Autodesk Inventor part; units mm, degrees
ref_plane "YZ Plane" through (0, 0, 0) normal (1, 0, 0) x (0, 1, 0)
ref_plane "XZ Plane" through (0, 0, 0) normal (0, 1, 0) x (-1, 0, 0)
ref_plane "XY Plane" through (0, 0, 0) normal (0, 0, 1) x (1, 0, 0)
sketch "Sketch1" plane through (0, 0, 0) normal (0, 0, 1) x (1, 0, 0)
  circle A0 centre (0, 0) radius 30
  dimension "d0" = 60
extrude "Extrusion1" add sketch "Sketch1" along normal mid plane 10
sketch "Sketch2" plane through (0, 0, 5) normal (0, 0, 1) x (1, 0, 0)
  circle A0 centre (0, 0) radius 30
  circle A1 centre (0, 0) radius 10
  dimension "d3" = 20
extrude "Extrusion2" add sketch "Sketch2" along normal blind 20 contours A1
sketch "Sketch3" plane through (0, 0, 25) normal (0, 0, 1) x (1, 0, 0)
  circle A0 centre (0, 0) radius 10
  circle A1 centre (0, 0) radius 5
  dimension "d6" = 10
extrude "Extrusion3" cut sketch "Sketch3" against normal through all contours A1
fillet "Fillet1" radius 3 1 edges at (-10, 0, 5)
chamfer "Chamfer1" distance 1 angle 45 1 edges at (-10, 0, 25)
sketch "Sketch5" plane through (0, 0, 5) normal (0, 0, 1) x (1, 0, 0)
  circle A0 centre (0, 0) radius 30
  circle A1 centre (0, 0) radius 5
  point P0 (-21, 0)
  point P1 (21, 0)
  point P2 (0, 22)
  point P3 (0, -22)
  dimension "d14" = 21
  dimension "d15" = 22
  dimension "d16" = 21
  dimension "d17" = 22
hole "Hole1" at (-21, 0, 5) at (21, 0, 5) at (0, 22, 5) at (0, -22, 5) direction (0, 0, -1) diameter 5 end through all
chamfer "Chamfer2" distance 0.5 angle 45 1 edges at (-30, 0, 5)
properties part number "Flange"
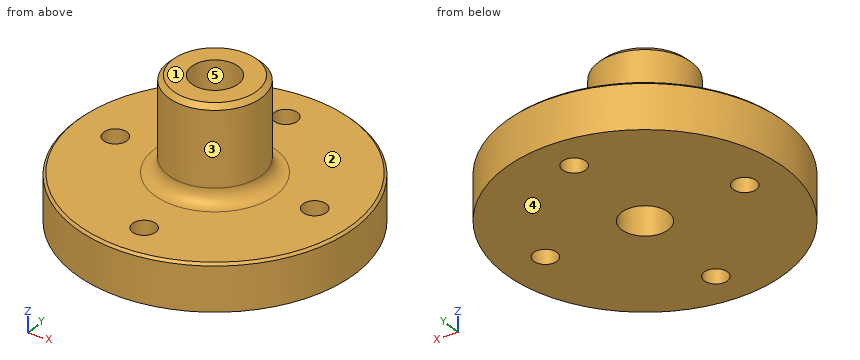
The model under review builds one solid part; all positions refer to its coordinate system, in mm. Face numbers are marked on the shaded views. A direction names the side the tool comes from. Give positions to 0.01 mm unless a question says otherwise; leave off trailing zeros. Order: outer loops, then holes, each group sorted by start corner. A loop starts at its lowest first (then second) coordinate and runs counter-clockwise, first axis right, second up. Notation, with made-up numbers: (81, 47) - (87, 47) arc R24 ccw to (87, 62) - close; hole circle Ø6 at (8, 24). An arc over 180 degrees is marked (long way). Use CSV: the item, a comma, the result in double quotes. Start each with the question number.
Q1. We need section C-C, the plane z = 15.25. Write out the cut boundary in (x, y), and give its area (3 significant figures).
Q2. To check wall thickness, follow line 1 along Y through (x, z) = (0, -0.75); line 2 along Z through (x, y) = (22, -18.5); line 3 along X through (y, z) = (-22, -1.25). State the ranges of each line that lie inside material, in increasing order. Write a range as [from, to].
Q3. We need section A-A, the plane y = 0. Write out the cut boundary in (x, z), and give its area (3 significant figures).
Q4. We need section B-B, the plane z = -3. Write out the cut boundary in (x, y).
Q5. Tool access review of the marked faces 1 and 2: name each direction out of +Z, -Z, +X, -X, +Y, -Y from which nothing blocks a thin tool from reaching the whole face with its end or side.
Q6. Clearance check with flat-ended pins moving along their axes: pin 1 Ø6 at (x, y) = (-18.5, 11) entering from +Z; pin 2 Ø4.5 at (x, y) = (21, 0) entering from -Z (3 decimals); pin 3 Ø5 at (y, z) = (-10.5, 19.5) entering from -X; pin 4 Ø12 at (y, z) = (-7, 1.5) entering from +X. State where each tip first meets the part, or that it passes through.
Q7. The part is to be moulded in two halves that separate along Y. For the marked faces 3, 4 and 5, say which applies: +Y half, -Y half, draft (parallel to the pull), parting line (faces both ways), or undercut.
Outcome:
1,outline,"circle Ø20 at (0, 0); hole circle Ø10 at (0, 0)"
1,area,"236 mm^2"
2,line 1,"y = [-30, -24.5], [-19.5, -5], [5, 19.5], [24.5, 30]"
2,line 2,"z = [-5, 5]"
2,line 3,"x = [-20.4, -2.5], [2.5, 20.4]"
3,outline,"(-30, -5) - (-23.5, -5) - (-23.5, 5) - (-29.5, 5) - (-30, 4.5) - close; (-18.5, -5) - (-5, -5) - (-5, 25) - (-9, 25) - (-10, 24) - (-10, 8) arc R3 cw to (-13, 5) - (-18.5, 5) - close; (5, -5) - (18.5, -5) - (18.5, 5) - (13, 5) arc R3 cw to (10, 8) - (10, 24) - (9, 25) - (5, 25) - close; (23.5, -5) - (30, -5) - (30, 4.5) - (29.5, 5) - (23.5, 5) - close"
3,area,"603 mm^2"
4,outline,"circle Ø60 at (0, 0); hole circle Ø5 at (-21, 0); hole circle Ø10 at (0, 0); hole circle Ø5 at (0, -22); hole circle Ø5 at (0, 22); hole circle Ø5 at (21, 0)"
5,face 1,"+Z, +X, -X, +Y, -Y"
5,face 2,"+Z"
6,pin 1,"stops at z = 5"
6,pin 2,"passes through"
6,pin 3,"stops at x = -6"
6,pin 4,"stops at x = 29.98"
7,face 3,"parting line"
7,face 4,"draft"
7,face 5,"undercut"
